Here's how the part is built. I have some questions about the finished solid (model axes, mm). A direction names the side the tool comes from. Round coordinates to 2 decimals unless told otherwise and drop trailing zeros. Order: outer loops, then holes, each group sorted by start corner. A loop starts at its lowest first (then second) coordinate and runs counter-clockwise, first axis right, second up. Notation, with made-up numbers: (57, -17.5) -> (78, -17.5) arc R15 ccw to (78, 4.5) -> close; hole circle Ø1 at (73.25, 36.5). An arc over 180 degrees is marked (long way). Answer in a Markdown table with one row per item.
```python
from build123d import *

# Parameters (mm, degrees)
F0_R     = 6.35
F1_DEPTH = 7
F2_R     = 3
F3_R     = 6.35
F3_R_2   = 3
F4_DEPTH = 4.8


with BuildPart() as f1:
    # F0 (on Top) → F1 (new body)
    with BuildSketch(Plane.XY):
        with BuildLine():
            Line((3.5, -24), (3.657538, -9.842378))
            ThreePointArc((3.657538, -9.842378), (-0.083786, 10.499666), (-3.5, -9.899495))
            Line((-3.5, -9.899495), (-3.5, -24))
            Line((-3.5, -24), (3.5, -24))
        make_face()
        Circle(F0_R, mode=Mode.SUBTRACT)
    extrude(amount=F1_DEPTH)

    # F2
    f2_edges = [f1.edges().sort_by_distance(p)[0] for p in [
        (-3.5, -9.899495, 3.5),
        (3.657538, -9.842378, 3.5),
    ]]
    fillet(f2_edges, radius=F2_R)

    # F3 (on face) → F4 (join)
    with BuildSketch(Plane(origin=(0, 0, 0), x_dir=(1, 0, 0), z_dir=(0, 0, -1))):
        Circle(F3_R)
        Circle(F3_R_2, mode=Mode.SUBTRACT)
    extrude(amount=-F4_DEPTH)


solid = f1.part
```
1. Suppose I cut it at D-D on x = 6. Write out the boundary of the cut face in (y, z).
Numbers:
| item | result |
|---|---|
| outline | (-8.62, 0) -> (8.62, 0) -> (8.62, 7) -> (2.08, 7) -> (2.08, 4.8) -> (-2.08, 4.8) -> (-2.08, 7) -> (-8.62, 7) -> close |
2. Suppose I cut it at B-B on z = 1.5. Write out the boundary of the cut face in (x, y), then the cut area to 3 significant figures.
Numbers:
| item | result |
|---|---|
| outline | (-5.06, -9.2) arc R3 cw to (-3.5, -11.83) -> (-3.5, -24) -> (3.5, -24) -> (3.64, -11.72) arc R3 cw to (5.16, -9.14) arc R10.5 ccw (long way) to start; hole circle Ø6 at (0, 0) |
| area | 416 mm2 |
3. For faces 1 (the face through (-3.5, -18, 3)), 2 (the face through (4.04, -10.25, 3.55)), which set-ups out of +Z, -Z, +X, -X, +Y, -Y let a thin tool reach every point of the face, with its end or its side?
Numbers:
| item | result |
|---|---|
| face 1 | +Z, -Z, -X, -Y |
| face 2 | +Z, -Z, +X, -Y |
4. Please list where these lines run through material, in increasing order: line 1 along Y through (x, z) = (0, 3.7); line 2 along X through (y, z) = (0, 3.6); line 3 along Y through (x, z) = (0, 5.9).
Numbers:
| item | result |
|---|---|
| line 1 | y = -24 to -3, 3 to 10.5 |
| line 2 | x = -10.5 to -3, 3 to 10.5 |
| line 3 | y = -24 to -6.35, 6.35 to 10.5 |
5. We'd pull the mould along Y, two halves only. Please class faces 3 (the face through (3, 1, 4.8)), 4 (the face through (-1.38, -6.2, 5.88)), 5 (the face through (-0.1, -3.2, 0)), 6 (the face through (0, -24, 3)): released by +Y, released by -Y, zero draft, split by the parting line, or undercut.
Numbers:
| item | result |
|---|---|
| face 3 | undercut |
| face 4 | undercut |
| face 5 | zero draft |
| face 6 | released by -Y |
6. Suppose I cut it at A-A on y = 0. Write out the boundary of the cut face in (x, z), then the cut area to 3 significant figures.
Numbers:
| item | result |
|---|---|
| outline | (-10.5, 0) -> (-3, 0) -> (-3, 4.8) -> (-6.35, 4.8) -> (-6.35, 7) -> (-10.5, 7) -> close; (3, 0) -> (10.5, 0) -> (10.5, 7) -> (6.35, 7) -> (6.35, 4.8) -> (3, 4.8) -> close |
| area | 90.3 mm2 |
7. Suppose I cut it at C-C on x = 0. Write out the boundary of the cut face in (y, z), then the cut area to 3 significant figures.
Numbers:
| item | result |
|---|---|
| outline | (-24, 0) -> (-3, 0) -> (-3, 4.8) -> (-6.35, 4.8) -> (-6.35, 7) -> (-24, 7) -> close; (3, 0) -> (10.5, 0) -> (10.5, 7) -> (6.35, 7) -> (6.35, 4.8) -> (3, 4.8) -> close |
| area | 185 mm2 |
8. For pin 1 Ø1 at (x, z) = (-1.5, 1.5) entering from +Y; pin 2 Ø3.5 at (y, z) = (-20, 4) entering from -X; pin 3 Ø1 at (y, z) = (-6.5, 1) entering from -X, each with a flat end and sliding along its axis, tell me the tip position at first contact or that it passes through.
Numbers:
| item | result |
|---|---|
| pin 1 | stops at y = 10.45 |
| pin 2 | stops at x = -3.5 |
| pin 3 | stops at x = -8.62 |
